```python
from build123d import *
from build123d.topology import SkipClean

# Parameters (mm, degrees)
SKETCH1_R           = 1
BOSS_EXTRUDE1_DEPTH = 10
SKETCH2_W           = 2
SKETCH2_H           = 3
SKETCH2_W_2         = 1
SKETCH2_H_2         = 2
SKETCH2_W_3         = 3
SKETCH2_H_3         = 1
CUT_EXTRUDE1_DEPTH  = 20
SKETCH3_W           = 11.356791525
SKETCH3_H           = 18.189557321
SKETCH3_R           = 3
CUT_EXTRUDE2_DEPTH  = 3
SKETCH4_R           = 2
CUT_EXTRUDE3_DEPTH  = 4
CUT_EXTRUDE4_START  = -2
CUT_EXTRUDE4_DEPTH  = 2
CUT_EXTRUDE5_START  = -2
SKETCH6_R           = 2
CUT_EXTRUDE5_DEPTH  = 2
SKETCH7_W           = 8
SKETCH7_H           = 4
CUT_EXTRUDE6_DEPTH  = 8
FILLET1_R           = 1
SKETCH9_R           = 1
CUT_EXTRUDE8_DEPTH  = 3
CUT_EXTRUDE9_DEPTH  = 9
CUT_EXTRUDE10_START = -4
SKETCH11_W          = 1
SKETCH11_H          = 2
SKETCH11_R          = 1
CUT_EXTRUDE10_DEPTH = 4
CUT_EXTRUDE11_DEPTH = 4
CUT_EXTRUDE12_DEPTH = 27
SKETCH14_R          = 1
CUT_EXTRUDE13_DEPTH = 27


with BuildPart() as part:
    # Sketch1 → Boss-Extrude1 (new body)
    with BuildSketch(Plane.XY):
        with BuildLine():
            Line((0, 0), (0, 14))
            Line((0, 14), (1, 14))
            ThreePointArc((1, 14), (2.171572875, 16.828427125), (5, 18))
            Line((5, 18), (10, 18))
            Line((10, 18), (18, 13))
            ThreePointArc((18, 13), (20, 9), (18, 5))
            Line((18, 5), (10, 0))
            Line((10, 0), (0, 0))
        make_face()
        with Locations((5, 14)):
            Circle(SKETCH1_R, mode=Mode.SUBTRACT)
        with Locations((15, 9)):
            Circle(SKETCH1_R, mode=Mode.SUBTRACT)
    extrude(amount=BOSS_EXTRUDE1_DEPTH)

    # Sketch2 → Cut-Extrude1 (cut)
    with BuildSketch(Plane(origin=(0, 18, 0), x_dir=(1, 0, 0), z_dir=(0, 1, 0))):
        Polygon((10, -7), (10, -10), (12, -10), (12, -9), (12, -7), align=None)
        with Locations((19, -8.5)):
            Rectangle(SKETCH2_W, SKETCH2_H)
        with Locations((19.5, -1)):
            Rectangle(SKETCH2_W_2, SKETCH2_H_2)
        with Locations((13.5, -9.5)):
            Rectangle(SKETCH2_W_3, SKETCH2_H_3)
    extrude(amount=-CUT_EXTRUDE1_DEPTH, mode=Mode.SUBTRACT)

    # Sketch3 → Cut-Extrude2 (cut)
    with BuildSketch(Plane.XY.offset(10)):
        with Locations((15.678395763, 9.094778661)):
            Rectangle(SKETCH3_W, SKETCH3_H)
        with Locations((15, 9)):
            Circle(SKETCH3_R, mode=Mode.SUBTRACT)
    extrude(amount=-CUT_EXTRUDE2_DEPTH, mode=Mode.SUBTRACT)

    # Sketch4 → Cut-Extrude3 (cut)
    with BuildSketch(Plane.XY.offset(10)):
        with Locations((15, 9)):
            Circle(SKETCH4_R)
    extrude(amount=-CUT_EXTRUDE3_DEPTH, mode=Mode.SUBTRACT)

    # Sketch5 → Cut-Extrude4 (cut)
    with BuildSketch(Plane(origin=(0, 0, 0), x_dir=(-1, 0, 0), z_dir=(0, 0, -1)).offset(CUT_EXTRUDE4_START)):
        with BuildLine():
            Line((-15, 6), (-23.076049943, 6))
            ThreePointArc((-23.076049943, 6), (-26.076049943, 9), (-23.076049943, 12))
            Line((-23.076049943, 12), (-15, 12))
            ThreePointArc((-15, 12), (-12, 9), (-15, 6))
        make_face()
    extrude(amount=CUT_EXTRUDE4_DEPTH, mode=Mode.SUBTRACT)

    # Sketch6 → Cut-Extrude5 (cut)
    with BuildSketch(Plane(origin=(0, 0, 2), x_dir=(-1, 0, 0), z_dir=(0, 0, -1)).offset(CUT_EXTRUDE5_START)):
        with Locations(Location((-15, 9, 0), (0, 0, 180))):
            Circle(SKETCH6_R)
    extrude(amount=CUT_EXTRUDE5_DEPTH, mode=Mode.SUBTRACT)

    # Sketch7 → Cut-Extrude6 (cut)
    with BuildSketch(Plane(origin=(0, 18, 0), x_dir=(1, 0, 0), z_dir=(0, 1, 0))):
        with Locations((5, -3)):
            Rectangle(SKETCH7_W, SKETCH7_H)
    extrude(amount=-CUT_EXTRUDE6_DEPTH, mode=Mode.SUBTRACT)

    # Fillet1
    fillet1_edges = [part.edges().sort_by_distance(p)[0] for p in [
        (1, 10, 3),
        (9, 10, 3),
    ]]
    fillet(fillet1_edges, radius=FILLET1_R)

    # Sketch9 → Cut-Extrude8 (cut)
    with BuildSketch(Plane(origin=(0, 10, 0), x_dir=(1, 0, 0), z_dir=(0, 1, 0))):
        with Locations(Location((7, -3, 0), (0, 0, 270))):
            Circle(SKETCH9_R)
        with Locations(Location((3, -3, 0), (0, 0, 270))):
            Circle(SKETCH9_R)
    extrude(amount=-CUT_EXTRUDE8_DEPTH, mode=Mode.SUBTRACT)

    # Sketch10 → Cut-Extrude9 (cut)
    with BuildSketch(Plane.XY.offset(10)):
        with BuildLine():
            Line((0, 7), (9, 7))
            ThreePointArc((9, 7), (9.707106781, 6.707106781), (10, 6))
            Line((10, 6), (10, 3))
            ThreePointArc((10, 3), (9.707106781, 2.292893219), (9, 2))
            Line((9, 2), (0, 2))
            Line((0, 2), (0, 7))
        make_face()
    extrude(amount=-CUT_EXTRUDE9_DEPTH, mode=Mode.SUBTRACT)

    # Sketch11 → Cut-Extrude10 (cut)
    # profile 1 of 3: a face of its own
    with BuildSketch(Plane.XY.offset(10).offset(CUT_EXTRUDE10_START)):
        with Locations((10.5, 11)):
            Rectangle(SKETCH11_W, SKETCH11_H)
    # profile 2 of 3: a face of its own
    with BuildSketch(Plane.XY.offset(10).offset(CUT_EXTRUDE10_START)):
        with Locations((10.5, 7)):
            Rectangle(SKETCH11_W, SKETCH11_H)
    # profile 3 of 3: a face of its own
    with BuildSketch(Plane.XY.offset(10).offset(CUT_EXTRUDE10_START)):
        with BuildLine():
            Line((1, 14), (0, 14))
            Line((0, 14), (0, 7))
            Line((0, 7), (9, 7))
            ThreePointArc((9, 7), (9.707106781, 6.707106781), (10, 6))
            Line((10, 6), (10, 18))
            Line((10, 18), (5, 18))
            ThreePointArc((5, 18), (2.171572875, 16.828427125), (1, 14))
        make_face()
        with Locations((5, 14)):
            Circle(SKETCH11_R, mode=Mode.SUBTRACT)
    extrude(amount=CUT_EXTRUDE10_DEPTH, mode=Mode.SUBTRACT)

    # Sketch12 → Cut-Extrude11 (cut)
    with BuildSketch(Plane.XY.offset(1)):
        with BuildLine():
            Line((2, 4), (-2.189178963, 4))
            ThreePointArc((-2.189178963, 4), (-3.189178963, 5), (-2.189178963, 6))
            Line((-2.189178963, 6), (2, 6))
            ThreePointArc((2, 6), (3, 5), (2, 4))
        make_face()
    extrude(amount=-CUT_EXTRUDE11_DEPTH, mode=Mode.SUBTRACT)

    # Sketch13 → Cut-Extrude12 (cut)
    with BuildSketch(Plane(origin=(0, 18, 0), x_dir=(1, 0, 0), z_dir=(0, 1, 0))):
        with BuildLine():
            Line((10, -9), (10, -10))
            Line((10, -10), (9, -10))
            ThreePointArc((9, -10), (9.707106781, -9.707106781), (10, -9))
        make_face()
        with BuildLine():
            Line((1, -10), (0, -10))
            Line((0, -10), (0, -9))
            ThreePointArc((0, -9), (0.292893219, -9.707106781), (1, -10))
        make_face()
    extrude(amount=-CUT_EXTRUDE12_DEPTH, mode=Mode.SUBTRACT)

    # Sketch14 → Cut-Extrude13 (cut)
    with BuildSketch(Plane(origin=(0, 2, 0), x_dir=(1, 0, 0), z_dir=(0, 1, 0))):
        with Locations(Location((5, -7, 0), (0, 0, 270))):
            Circle(SKETCH14_R)
    extrude(amount=-CUT_EXTRUDE13_DEPTH, mode=Mode.SUBTRACT)

    # Sketch15 → Revolve1 (revolve)
    with BuildSketch(Plane.XY.offset(7)):
        with BuildLine():
            Line((4, 2), (4, 2.5))
            ThreePointArc((4, 2.5), (3.853553391, 2.146446609), (3.5, 2))
            Line((3.5, 2), (4, 2))
        make_face()
    revolve(axis=Axis((5, 0, 7), (0, 1, 0)))

    # Sketch16 → Revolve2 (revolve)
    with SkipClean():  # the faces are left unmerged after this step: merging them gives an invalid solid
        with BuildSketch(Plane(origin=(0, 14, 0), x_dir=(1, 0, 0), z_dir=(0, 1, 0))):
            with BuildLine():
                Line((4, -6), (4, -6.5))
                ThreePointArc((4, -6.5), (3.853553391, -6.146446609), (3.5, -6))
                Line((3.5, -6), (4, -6))
            make_face()
        revolve(axis=Axis((5, 14, 5), (0, 0, 1)))
    add(part.part.scale(1), mode=Mode.REPLACE)  # the faces are merged on a copy


solid = part.part
```
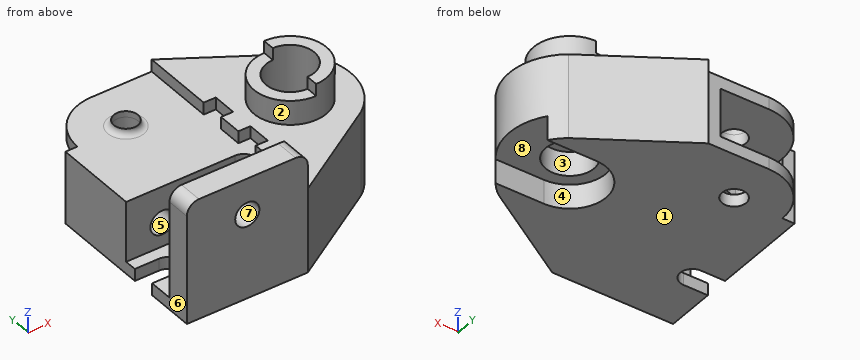
Work out the finished part from the listing and answer in its coordinate system (mm). Face numbers are marked on the shaded views. A direction names the side the tool comes from. Give positions to 0.01 mm unless a question says otherwise; leave off trailing zeros. Write each loop counter-clockwise with the first axis right and the second up, starting at its lowest first coordinate (ties: lowest second). Pieces come first, ordered by that corner, then holes.
(1) The part is cut by section D-D on z = 7.75. Count the separate pieces of the cut face and the enclosed holes in it, plus the area to 3 significant figures.
Final values:
separate pieces: 3
enclosed holes: 1
area: 33.4 mm2
(2) Straight lines are drawn through the part: line 1 (Z direction, x = 1.5, y = 14.75); line 2 (X direction, y = 9, z = 5.6); line 3 (X direction, y = 8, z = 3). For each, find the intervals that lie inside material, in ascending order.
Final values:
line 1: z = 0 to 1, 5 to 6
line 2: x = 0 to 14, 16 to 20
line 3: x = 0 to 2, 4 to 6, 8 to 13.27, 16.73 to 19.9
(3) The part is cut by section A-A on y = 9. Write down the section's boundary in (x, z), plus the area to 3 significant figures.
Final values:
outline: (0, 0) - (12, 0) - (12, 2) - (13, 2) - (13, 4) - (14, 4) - (14, 6) - (13, 6) - (13, 9) - (12, 9) - (12, 7) - (10, 7) - (10, 6) - (0, 6) - close; (16, 4) - (17, 4) - (17, 2) - (20, 2) - (20, 7) - (18, 7) - (18, 10) - (17, 10) - (17, 6) - (16, 6) - close; hole circle Ø2 at (3, 3); hole circle Ø2 at (7, 3)
area: 96.7 mm2
(4) The part is cut by section B-B on y = 1.25. Write down the section's boundary in (x, z).
Final values:
outline: (0, 0) - (12, 0) - (12, 7) - (10, 7) - (10, 9) arc R1 ccw to (9, 10) - (1, 10) arc R1 ccw to (0, 9) - close; hole circle Ø2 at (5, 7)
(5) The mould has two halves that part along Z. Classify the marked faces 6, 7 and 8: pulls with the +Z half, pulls with the -Z half, needs draft (parallel to the pull), parting line crosses it, or undercut.
Final values:
face 6: needs draft
face 7: undercut
face 8: pulls with the -Z half
(6) Which of the six approach directions +Z, -Z, +X, -X, +Y, -Y give full straight-line access (tool end or side, diameter ignored) to the marked faces 1, 2, 3, 4 and 5?
Final values:
face 1: -Z, +X, -X, +Y, -Y
face 2: +Z
face 3: -Z
face 4: -Z, +X
face 5: +Y
(7) Flat-ended cylindrical pins translate along their axes: pin 1 Ø8 at (x, y) = (13, 5) entering from +Z; pin 2 Ø0.5 at (y, z) = (11, 6.5) entering from -X; pin 3 Ø1.5 at (x, z) = (8, 2) entering from +Y; pin 4 Ø3.5 at (y, z) = (13, 3) entering from +X. Find the tip coordinate at first contact, or state that the pin passes through.
Final values:
pin 1: stops at z = 10
pin 2: stops at x = 11
pin 3: stops at y = 10.34
pin 4: stops at x = 19.47
(8) The part is cut by section C-C on x = 15.75. Write down the section's boundary in (y, z).
Final values:
outline: (3.59, 0) - (6, 0) - (6, 2) - (7.15, 2) - (7.15, 4) - (8.34, 4) - (8.34, 6) - (7.15, 6) - (7.15, 10) - (6.1, 10) - (6.1, 7) - (3.59, 7) - close; (9.66, 4) - (10.85, 4) - (10.85, 2) - (12, 2) - (12, 0) - (14.41, 0) - (14.41, 7) - (11.9, 7) - (11.9, 10) - (10.85, 10) - (10.85, 6) - (9.66, 6) - close
